Check sheet for the modelled part. Datum: model origin and axes. Units: mm. Face numbers are marked on the shaded views. A direction names the side the tool comes from. Round coordinates to 2 decimals unless told otherwise and drop trailing zeros. Loops run counter-clockwise (first coordinate to the right, second up) from the corner with the lowest first, then second, coordinate; pieces in that order, holes last. Notation, with made-up numbers: (-9.75, 8.5) - (20.25, 8.5) arc R29 cw to (20.25, 47.5) - close; hole circle Ø6 at (61.25, -23.75). An arc over 180 degrees is marked (long way). Put each result on its own line as item: value. Start each with the question number.
Item 1: Tool access check on the marked faces 1, 2 and 3. Record the directions out of +Z, -Z, +X, -X, +Y, -Y that give a thin tool (end or side, any length) a straight path to the whole face; none if there is none.
Item 2: Section check B-B, the plane z = 13.75. Record the cut outline in (x, y).
Item 3: Section check C-C, the plane z = 19. Record the cut outline in (x, y).
Item 4: Gauge pin test, flat ends, axial feed: pin 1 Ø2.5 at (x, z) = (-13.93, 11.11) entering from -Y; pin 2 Ø1 at (y, z) = (2, 19.5) entering from +X. Record the tip position at first contact, or that the pin passes through.
Item 5: Section check D-D, the plane x = -13.75. Give the number of separate pieces and of enclosed holes in the cut face, and give its area (3 significant figures).
Item 6: Material ranges on line 1 along X through (y, z) = (2, 7.75); line 2 along X through (y, z) = (0.1, 12.5); line 3 along X through (y, z) = (2.6, 14.25), recorded low to high.
Item 7: Section check A-A, the plane x = -16.5. Record the cut outline in (y, z).
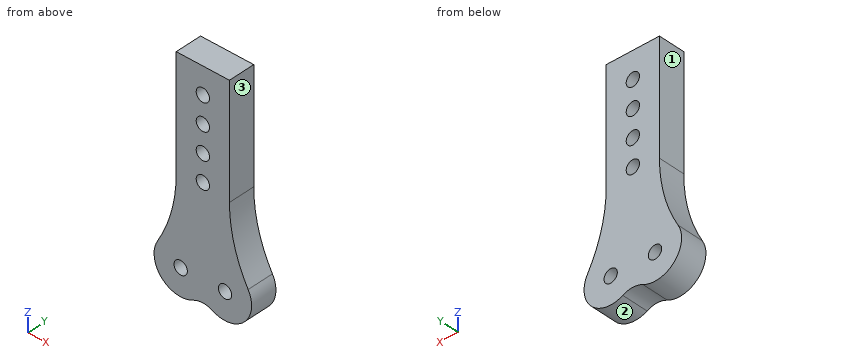
from build123d import *

# Parameters (mm, degrees)
CROQUIS2_W              = 6
CROQUIS2_H              = 22
SALIENTE_EXTRUIR2_DEPTH = 3
CROQUIS7_R              = 3
SALIENTE_EXTRUIR4_DEPTH = 3
REDONDEO2_R             = 2.5
CROQUIS11_R             = 0.75
CORTAR_EXTRUIR6_DEPTH   = 3
CROQUIS12_R             = 0.75
CORTAR_EXTRUIR7_DEPTH   = 10
REDONDEO3_R             = 16


with BuildPart() as part:
    # Croquis2 → Saliente-Extruir2 (new body)
    with BuildSketch(Plane(origin=(0, 0, 0), x_dir=(1, 0, 0), z_dir=(0, 1, 0))):
        with Locations((-13.931432693, -12.112220068)):
            Rectangle(CROQUIS2_W, CROQUIS2_H)
    extrude(amount=SALIENTE_EXTRUIR2_DEPTH)

    # Croquis7 → Saliente-Extruir4 (add)
    with BuildSketch(Plane(origin=(0, 3, 0), x_dir=(1, 0, 0), z_dir=(0, 1, 0))):
        with Locations((-16.431432693, -1.112220068)):
            Circle(CROQUIS7_R)
        with Locations((-11.431432693, -1.112220068)):
            Circle(CROQUIS7_R)
    extrude(amount=-SALIENTE_EXTRUIR4_DEPTH)

    # Redondeo2
    redondeo2_edges = [part.edges().sort_by_distance(p)[0] for p in [
        (-13.931432693, 1.5, -0.546092328),
    ]]
    fillet(redondeo2_edges, radius=REDONDEO2_R)

    # Croquis11 → Cortar-Extruir6 (cut)
    with BuildSketch(Plane(origin=(0, 3, 0), x_dir=(1, 0, 0), z_dir=(0, 1, 0))):
        with Locations((-16.431432693, -1.112220068)):
            Circle(CROQUIS11_R)
        with Locations((-11.431432693, -1.112220068)):
            Circle(CROQUIS11_R)
    extrude(amount=-CORTAR_EXTRUIR6_DEPTH, mode=Mode.SUBTRACT)

    # Croquis12 → Cortar-Extruir7 (cut)
    with BuildSketch(Plane.XZ):
        with Locations((-13.931432693, 20.112220068)):
            Circle(CROQUIS12_R)
        with Locations((-13.931432693, 17.112220068)):
            Circle(CROQUIS12_R)
        with Locations((-13.931432693, 14.112220068)):
            Circle(CROQUIS12_R)
        with Locations((-13.931432693, 11.112220068)):
            Circle(CROQUIS12_R)
    extrude(amount=-CORTAR_EXTRUIR7_DEPTH, mode=Mode.SUBTRACT)

    # Redondeo3
    redondeo3_edges = [part.edges().sort_by_distance(p)[0] for p in [
        (-10.931432693, 1.5, 4.070259959),
        (-16.931432693, 1.5, 4.070259959),
    ]]
    fillet(redondeo3_edges, radius=REDONDEO3_R)


solid = part.part
Check result:
1. face 1: +Z, -X, +Y, -Y
1. face 2: +Y, -Y
1. face 3: +Z, +X, +Y, -Y
2. outline: (-16.93, 0) - (-14.59, 0) - (-14.59, 3) - (-16.93, 3) - close; (-13.27, 0) - (-10.93, 0) - (-10.93, 3) - (-13.27, 3) - close
3. outline: (-16.93, 0) - (-10.93, 0) - (-10.93, 3) - (-16.93, 3) - close
4. pin 1: y = 0
4. pin 2: x = -10.93
5. separate pieces: 5
5. enclosed holes: 0
5. area: 55.8 mm²
6. line 1: -17.18 to -10.69
6. line 2: -16.93 to -10.93
6. line 3: -16.93 to -14.67, -13.19 to -10.93
7. outline: (0, -1.89) - (3, -1.89) - (3, 0.37) - (0, 0.37) - close; (0, 1.86) - (3, 1.86) - (3, 23.11) - (0, 23.11) - close
